Check sheet for the modelled part. Datum: model origin and axes. Units: mm. Give positions to 0.01 mm unless a question says otherwise; leave off trailing zeros. Loops run counter-clockwise (first coordinate to the right, second up) from the corner with the lowest first, then second, coordinate; pieces in that order, holes last. Notation, with made-up numbers: (-26.75, -19) - (-6.75, -19) arc R35 cw to (-6.75, 14) - close; hole circle Ø9 at (-16.75, 80). An arc over 180 degrees is marked (long way). Use CSV: the item, a comma, the result in double quotes.
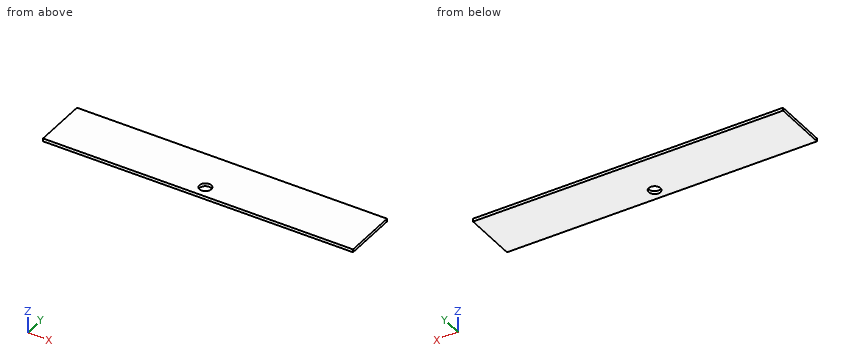
from build123d import *

# Parameters (mm, degrees)
SKETCH1_W           = 660.4
SKETCH1_H           = 115
BOSS_EXTRUDE1_DEPTH = 6.35
SKETCH2_R           = 12.5
CUT_EXTRUDE1_DEPTH  = 343.304487993


with BuildPart() as part:
    # Sketch1 → Boss-Extrude1 (new body)
    with BuildSketch(Plane.XY):
        with Locations((0, 32.5)):
            Rectangle(SKETCH1_W, SKETCH1_H)
    extrude(amount=BOSS_EXTRUDE1_DEPTH)

    # Sketch2 → Cut-Extrude1 (cut, through all)
    with BuildSketch(Plane(origin=(0, 0, 0), x_dir=(-1, 0, 0), z_dir=(0, 0, -1))):
        Circle(SKETCH2_R)
    extrude(amount=-CUT_EXTRUDE1_DEPTH, mode=Mode.SUBTRACT)


solid = part.part
1. Scan lines: line 1 along Y through (x, z) = (0, 3.75); line 2 along X through (y, z) = (-6, 6). Record each from-to range of solid material in increasing order.
Completed:
line 1,"y = -25 to -12.5, 12.5 to 90"
line 2,"x = -330.2 to -10.97, 10.97 to 330.2"
2. Sectioned sample at A-A, the plane y = 0. Record the boundary of the cut face in (x, z), and give its area (3 significant figures).
Completed:
outline,"(-330.2, 0) - (-12.5, 0) - (-12.5, 6.35) - (-330.2, 6.35) - close; (12.5, 0) - (330.2, 0) - (330.2, 6.35) - (12.5, 6.35) - close"
area,"4,030 mm²"
3. Sectioned sample at B-B, the plane x = 0. Record the boundary of the cut face in (y, z).
Completed:
outline,"(-25, 0) - (-12.5, 0) - (-12.5, 6.35) - (-25, 6.35) - close; (12.5, 0) - (90, 0) - (90, 6.35) - (12.5, 6.35) - close"
